Source: CAD feature listing. Evaluate the final solid. Frame: model axes, mm. A direction names the side the tool comes from. Coordinates: 2 decimals unless noted, no trailing zeros. Write each loop counter-clockwise with the first axis right and the second up, starting at its lowest first coordinate (ties: lowest second). Pieces come first, ordered by that corner, then holes. Notation, with made-up numbers: (81, 60.5) -> (100, 60.5) arc R31 ccw to (100, 90.5) -> close; hole circle Ø1 at (-14.5, 35). An arc over 180 degrees is marked (long way). One line per item, written item: value. Start each with the question number.
1. Mould query, pull axis Y, two halves, no side actions, for faces 3 (the cylindrical face through (1.52, 24.55, -15.3)), 4 (the cylindrical face through (1.52, -24.26, -8.07)), 5 (the flat face through (4, 11, 16)), 6 (the flat face through (1.1, -18, 13)). Classes: released by +Y, released by -Y, zero draft, split by the parting line, or undercut.
2. Access query for faces 1 (the cylindrical face through (2.57, 21.6, -13.21)), 2 (the cylindrical face through (1.521, 24.263, -8.209)). Directions: +Z, -Z, +X, -X, +Y, -Y. A direction counts if a zero-diameter tool reaches every point of the face in a straight line with its end or side. Return the directions, or none.
3. First-contact query: P1, Ø3, axis at y = 19.21, z = -13.96, coming from the +X side; P2, Ø1.5, axis at y = -14, z = -19, coming from the +X side; P3, Ø1, axis at x = 1.5, y = 5.5, coming from the +Z side; P4, Ø1, axis at x = 1.5, z = -9, coming from the -Y side. Flat tips, straight axial feed; report the tip coordinate or a pass-through.
4. Line query: line 1 (X direction, y = -14, z = 9); line 2 (Y direction, x = 2.8, z = -13); line 3 (Y direction, x = -0.15, z = -14.5). Output: solid intervals per line, ascending.
5. Section query A-A, the plane y = 0. Output: boundary loops of the cut face in (x, z).
from build123d import *

# Parameters (mm, degrees)
SKETCH_1_R                     = 30
EXTRUDE_1_DEPTH                = 4
EXTRUDE_2_DEPTH                = 1.9
CHAMFER_1_SIZE                 = 1
SKETCH_5_R                     = 16
CUT_EXTRUDE_2_DEPTH            = 43.83468221
HOLE_WIZARD_M2_5_1_D           = 2.7
HOLE_WIZARD_M2_5_1_CBORE_D     = 5
HOLE_WIZARD_M2_5_1_CBORE_DEPTH = 2.9
SKETCH_8_OUTSIDE_W             = 79.012
SKETCH_8_OUTSIDE_H             = 79.012
CUT_EXTRUDE_3_DEPTH            = 43.83468221
CHAMFER_2_SIZE                 = 1
SKETCH_9_R                     = 18.55
CUT_EXTRUDE_4_DEPTH            = 2.5
CHAMFER_3_SIZE                 = 0.5


with BuildPart() as part:
    # 草图1 → 凸台-拉伸1 (new body)
    with BuildSketch(Plane.YZ):
        with Locations(Location((0, 0, 0), (0, 0, 270))):
            Circle(SKETCH_1_R)
    extrude(amount=EXTRUDE_1_DEPTH)

    # 草图2 → 凸台-拉伸2 (add)
    with BuildSketch(Plane(origin=(0, 0, 0), x_dir=(0, -1, 0), z_dir=(-1, 0, 0))):
        with BuildLine():
            ThreePointArc((-15.429362873, -21.236696102), (-14.556584324, -21.641903091), (-13.595407183, -21.687439927))
            ThreePointArc((-13.595407183, -21.687439927), (-8.168716079, -21.262073185), (-2.734521388, -21.577416267))
            ThreePointArc((-2.734521388, -21.577416267), (0, -21.75), (2.734521388, -21.577416267))
            ThreePointArc((2.734521388, -21.577416267), (8.168716079, -21.262073185), (13.595407183, -21.687439927))
            ThreePointArc((13.595407183, -21.687439927), (14.556584324, -21.641903091), (15.429362873, -21.236696102))
            ThreePointArc((15.429362873, -21.236696102), (18.561553006, -18.561553006), (21.236696102, -15.429362873))
            ThreePointArc((21.236696102, -15.429362873), (21.641903091, -14.556584324), (21.687439927, -13.595407183))
            ThreePointArc((21.687439927, -13.595407183), (21.262073185, -8.168716079), (21.577416267, -2.734521388))
            ThreePointArc((21.577416267, -2.734521388), (21.75, 0), (21.577416267, 2.734521388))
            ThreePointArc((21.577416267, 2.734521388), (21.262073185, 8.168716079), (21.687439927, 13.595407183))
            ThreePointArc((21.687439927, 13.595407183), (21.641903091, 14.556584324), (21.236696102, 15.429362873))
            ThreePointArc((21.236696102, 15.429362873), (18.561553006, 18.561553006), (15.429362873, 21.236696102))
            ThreePointArc((15.429362873, 21.236696102), (14.556584324, 21.641903091), (13.595407183, 21.687439927))
            ThreePointArc((13.595407183, 21.687439927), (8.168716079, 21.262073185), (2.734521388, 21.577416267))
            ThreePointArc((2.734521388, 21.577416267), (0, 21.75), (-2.734521388, 21.577416267))
            ThreePointArc((-2.734521388, 21.577416267), (-8.168716079, 21.262073185), (-13.595407183, 21.687439927))
            ThreePointArc((-13.595407183, 21.687439927), (-14.556584324, 21.641903091), (-15.429362873, 21.236696102))
            ThreePointArc((-15.429362873, 21.236696102), (-18.561553006, 18.561553006), (-21.236696102, 15.429362873))
            ThreePointArc((-21.236696102, 15.429362873), (-21.641903091, 14.556584324), (-21.687439927, 13.595407183))
            ThreePointArc((-21.687439927, 13.595407183), (-21.262073185, 8.168716079), (-21.577416267, 2.734521388))
            ThreePointArc((-21.577416267, 2.734521388), (-21.75, 0), (-21.577416267, -2.734521388))
            ThreePointArc((-21.577416267, -2.734521388), (-21.262073185, -8.168716079), (-21.687439927, -13.595407183))
            ThreePointArc((-21.687439927, -13.595407183), (-21.641903091, -14.556584324), (-21.236696102, -15.429362873))
            ThreePointArc((-21.236696102, -15.429362873), (-18.561553006, -18.561553006), (-15.429362873, -21.236696102))
        make_face()
    extrude(amount=EXTRUDE_2_DEPTH)

    # 倒角1
    chamfer_1_edges = [part.edges().sort_by_distance(p)[0] for p in [
        (0, 21.641903091, -14.556584324),
        (0, 18.561553006, -18.561553006),
        (0, 14.556584324, -21.641903091),
        (0, 8.168716079, -21.262073185),
        (0, 0, -21.75),
        (0, -8.168716079, -21.262073185),
        (0, -14.556584324, -21.641903091),
        (0, -18.561553006, -18.561553006),
        (0, -21.641903091, -14.556584324),
        (0, -21.262073185, -8.168716079),
        (0, -21.75, 0),
        (0, -21.262073185, 8.168716079),
        (0, -21.641903091, 14.556584324),
        (0, -18.561553006, 18.561553006),
        (0, -14.556584324, 21.641903091),
        (0, -8.168716079, 21.262073185),
        (0, 0, 21.75),
        (0, 8.168716079, 21.262073185),
        (0, 14.556584324, 21.641903091),
        (0, 18.561553006, 18.561553006),
        (0, 21.641903091, 14.556584324),
        (0, 21.262073185, 8.168716079),
        (0, 21.75, 0),
        (0, 21.262073185, -8.168716079),
    ]]
    chamfer(chamfer_1_edges, length=CHAMFER_1_SIZE)

    # 草图5 → 切除-拉伸2 (cut, through all)
    with BuildSketch(Plane.YZ.offset(4)):
        with Locations(Location((0, 0, 0), (0, 0, 270))):
            Circle(SKETCH_5_R)
    extrude(amount=-CUT_EXTRUDE_2_DEPTH, mode=Mode.SUBTRACT)

    # M2.5 六角圆柱头螺钉的柱形沉头孔1 (through all)
    with Locations(Plane.YZ.offset(4)):
        with Locations((-19.214153616, 13.959899742), (13.959899742, 19.214153616), (19.214153616, -13.959899742), (-13.959899742, -19.214153616)):
            CounterBoreHole(HOLE_WIZARD_M2_5_1_D / 2, HOLE_WIZARD_M2_5_1_CBORE_D / 2, HOLE_WIZARD_M2_5_1_CBORE_DEPTH)

    # 草图8 outside → 切除-拉伸3 (cut, through all)
    with BuildSketch(Plane(origin=(4, 0, 0), x_dir=(0, 0, -1), z_dir=(1, 0, 0))):
        Rectangle(SKETCH_8_OUTSIDE_W, SKETCH_8_OUTSIDE_H)
        with BuildLine():
            ThreePointArc((-3.111696751, 24.553611615), (-8.138326841, 24.261919263), (-13.158016112, 24.6553835))
            ThreePointArc((-13.158016112, 24.6553835), (-15.272605822, 24.55520246), (-17.19271863, 23.663747085))
            ThreePointArc((-17.19271863, 23.663747085), (-20.68287335, 20.68287335), (-23.663747085, 17.19271863))
            ThreePointArc((-23.663747085, 17.19271863), (-24.55520246, 15.272605822), (-24.6553835, 13.158016112))
            ThreePointArc((-24.6553835, 13.158016112), (-24.261919263, 8.138326841), (-24.553611615, 3.111696751))
            ThreePointArc((-24.553611615, 3.111696751), (-24.75, 0), (-24.553611615, -3.111696751))
            ThreePointArc((-24.553611615, -3.111696751), (-24.261919263, -8.138326841), (-24.6553835, -13.158016112))
            ThreePointArc((-24.6553835, -13.158016112), (-24.55520246, -15.272605822), (-23.663747085, -17.19271863))
            ThreePointArc((-23.663747085, -17.19271863), (-20.68287335, -20.68287335), (-17.19271863, -23.663747085))
            ThreePointArc((-17.19271863, -23.663747085), (-15.272605822, -24.55520246), (-13.158016112, -24.6553835))
            ThreePointArc((-13.158016112, -24.6553835), (-8.138326841, -24.261919263), (-3.111696751, -24.553611615))
            ThreePointArc((-3.111696751, -24.553611615), (0, -24.75), (3.111696751, -24.553611615))
            ThreePointArc((3.111696751, -24.553611615), (8.138326841, -24.261919263), (13.158016112, -24.6553835))
            ThreePointArc((13.158016112, -24.6553835), (15.272605822, -24.55520246), (17.19271863, -23.663747085))
            ThreePointArc((17.19271863, -23.663747085), (20.68287335, -20.68287335), (23.663747085, -17.19271863))
            ThreePointArc((23.663747085, -17.19271863), (24.55520246, -15.272605822), (24.6553835, -13.158016112))
            ThreePointArc((24.6553835, -13.158016112), (24.261919263, -8.138326841), (24.553611615, -3.111696751))
            ThreePointArc((24.553611615, -3.111696751), (24.75, 0), (24.553611615, 3.111696751))
            ThreePointArc((24.553611615, 3.111696751), (24.261919263, 8.138326841), (24.6553835, 13.158016112))
            ThreePointArc((24.6553835, 13.158016112), (24.55520246, 15.272605822), (23.663747085, 17.19271863))
            ThreePointArc((23.663747085, 17.19271863), (20.68287335, 20.68287335), (17.19271863, 23.663747085))
            ThreePointArc((17.19271863, 23.663747085), (15.272605822, 24.55520246), (13.158016112, 24.6553835))
            ThreePointArc((13.158016112, 24.6553835), (8.138326841, 24.261919263), (3.111696751, 24.553611615))
            ThreePointArc((3.111696751, 24.553611615), (0, 24.75), (-3.111696751, 24.553611615))
        make_face(mode=Mode.SUBTRACT)
    extrude(amount=-CUT_EXTRUDE_3_DEPTH, mode=Mode.SUBTRACT)

    # 倒角2
    chamfer_2_edges = [part.edges().sort_by_distance(p)[0] for p in [
        (4, 24.75, 0),
        (4, 24.261919263, -8.138326841),
        (4, 24.55520246, -15.272605822),
        (4, 20.68287335, -20.68287335),
        (4, 15.272605822, -24.55520246),
        (4, 8.138326841, -24.261919263),
        (4, 0, -24.75),
        (4, -8.138326841, -24.261919263),
        (4, -15.272605822, -24.55520246),
        (4, -20.68287335, -20.68287335),
        (4, -24.55520246, -15.272605822),
        (4, -24.261919263, -8.138326841),
        (4, -24.75, 0),
        (4, -24.261919263, 8.138326841),
        (4, -24.55520246, 15.272605822),
        (4, -20.68287335, 20.68287335),
        (4, -15.272605822, 24.55520246),
        (4, -8.138326841, 24.261919263),
        (4, 0, 24.75),
        (4, 8.138326841, 24.261919263),
        (4, 15.272605822, 24.55520246),
        (4, 20.68287335, 20.68287335),
        (4, 24.55520246, 15.272605822),
        (4, 24.261919263, 8.138326841),
    ]]
    chamfer(chamfer_2_edges, length=CHAMFER_2_SIZE)

    # 草图9 → 切除-拉伸4 (cut)
    with BuildSketch(Plane(origin=(4, 0, 0), x_dir=(0, 0, -1), z_dir=(1, 0, 0))):
        Circle(SKETCH_9_R)
    extrude(amount=-CUT_EXTRUDE_4_DEPTH, mode=Mode.SUBTRACT)

    # 倒角3
    chamfer_3_edges = [part.edges().sort_by_distance(p)[0] for p in [
        (-1.9, 0, 16),
        (1.5, 0, 16),
    ]]
    chamfer(chamfer_3_edges, length=CHAMFER_3_SIZE)


solid = part.part
Computed values:
1. face 3: released by +Y
1. face 4: released by -Y
1. face 5: zero draft
1. face 6: undercut
2. face 1: +X
2. face 2: +X, -X, +Y
3. P1: stops at x = 1.1
3. P2: passes through
3. P3: stops at z = 24.36
3. P4: stops at y = -24.3
4. line 1: x = -1.9 to 1.5
4. line 2: y = -24.63 to -13.23, 13.23 to 16.91, 21.52 to 24.63
4. line 3: y = -22.52 to -6.76, 6.76 to 17.98, 20.45 to 22.52
5. outline: (-1.9, -21.75) -> (-1, -21.75) -> (0, -22.75) -> (0, -24.75) -> (3, -24.75) -> (4, -23.75) -> (4, -18.55) -> (1.5, -18.55) -> (1.5, -16.5) -> (1, -16) -> (-1.4, -16) -> (-1.9, -16.5) -> close; (-1.9, 16.5) -> (-1.4, 16) -> (1, 16) -> (1.5, 16.5) -> (1.5, 18.55) -> (4, 18.55) -> (4, 23.75) -> (3, 24.75) -> (0, 24.75) -> (0, 22.75) -> (-1, 21.75) -> (-1.9, 21.75) -> close
